Source: CAD feature listing. Evaluate the final solid. Frame: model axes, mm. Give positions to 0.01 mm unless a question says otherwise; leave off trailing zeros. Order: outer loops, then holes, each group sorted by start corner. A loop starts at its lowest first (then second) coordinate and runs counter-clockwise, first axis right, second up.
```python
from build123d import *

# Parameters (mm, degrees)
SKETCH1_W           = 8
SKETCH1_H           = 3.5
BOSS_EXTRUDE1_DEPTH = 5
SKETCH2_W           = 8
SKETCH2_H           = 3.5
BOSS_EXTRUDE2_DEPTH = 8
CHAMFER1_SIZE       = 0.5


with BuildPart() as part:
    # Sketch1 → Boss-Extrude1 (new, symmetric)
    with BuildSketch(Plane.XY):
        Rectangle(SKETCH1_W, SKETCH1_H)
    extrude(amount=BOSS_EXTRUDE1_DEPTH, both=True)

    # Sketch2 → Boss-Extrude2 (add)
    with BuildSketch(Plane(origin=(0, 0, -5), x_dir=(-1, 0, 0), z_dir=(0, 0, -1))):
        Rectangle(SKETCH2_W, SKETCH2_H)
    boss_extrude2 = extrude(amount=BOSS_EXTRUDE2_DEPTH)

    # Mirror1: Boss-Extrude2 across plane
    add(boss_extrude2.mirror(Plane.XY))

    # Chamfer1
    chamfer1_edges = [part.edges().sort_by_distance(p)[0] for p in [
        (-4, 0, -13),
        (0, 1.75, -13),
        (4, 0, -13),
        (0, -1.75, -13),
        (-4, 0, 13),
        (0, -1.75, 13),
        (4, 0, 13),
        (0, 1.75, 13),
        (4, -1.75, 0),
        (-4, -1.75, 0),
        (-4, 1.75, 0),
        (4, 1.75, 0),
    ]]
    chamfer(chamfer1_edges, length=CHAMFER1_SIZE)


solid = part.part
```
1) Draft query along Y for faces 1 (the flat face through (0, 1.75, 0)), 2 (the flat face through (0, 0, -13)), 3 (the flat face through (0, -1.75, 0)). Return one class per face: +Y half, -Y half, draft (parallel to the pull), parting line (faces both ways), or undercut.
Report:
face 1: +Y half
face 2: draft
face 3: -Y half
2) Material intervals for L1, parallel to Z at x = 2.5, y = -1.4; L2, parallel to X at y = 1.3, z = -7; L3, parallel to Y at x = 3.75, z = -9.75, sorted ascending.
Report:
L1: z = -12.85 to 12.85
L2: x = -3.95 to 3.95
L3: y = -1.5 to 1.5
3) Section query A-A, the plane z = 6. Return the cut outline in (x, y).
Report:
outline: (-4, -1.25) - (-3.5, -1.75) - (3.5, -1.75) - (4, -1.25) - (4, 1.25) - (3.5, 1.75) - (-3.5, 1.75) - (-4, 1.25) - close
